The model under review builds one solid part; all positions refer to its coordinate system, in mm. A direction names the side the tool comes from. Give positions to 0.01 mm unless a question says otherwise; leave off trailing zeros. Loops run counter-clockwise (first coordinate to the right, second up) from the corner with the lowest first, then second, coordinate; pieces in that order, holes last. Notation, with made-up numbers: M -6.75,-23 L 51.25,-23 A19 ccw 51.25,-2 Z; hole C -5.5,-29 d4. An arc over 180 degrees is marked long. Return JSON: item names as keys, results as strings. Group by question number.
```python
from build123d import *

# Parameters (mm, degrees)
SKETCH1_W           = 7.9375
SKETCH1_H           = 360.02418597
SKETCH1_3_R         = 12.7
BOSS_EXTRUDE1_DEPTH = 1.5875
SCALE1_SCALE        = 0.5


with BuildPart() as part:
    # Sketch1 → Revolve1 (revolve)
    with BuildSketch(Plane.XY, mode=Mode.PRIVATE) as revolve1_sk:
        with Locations((3.96875, 206.8008909)):
            Rectangle(SKETCH1_W, SKETCH1_H)
    revolve(revolve1_sk.sketch.rotate(Axis((0, 386.812983885, 0), (0, -1, 0)), 180), axis=Axis((0, 386.812983885, 0), (0, -1, 0)))

    # Sketch1_3 → Boss-Extrude1 (add, symmetric)
    # profile 1 of 2: a face of its own
    with BuildSketch(Plane.XY):
        with BuildLine():
            Line((-7.9375, 26.788797915), (7.9375, 26.788797915))
            ThreePointArc((7.9375, 26.788797915), (0, -27.94), (-7.9375, 26.788797915))
        make_face()
        Circle(SKETCH1_3_R, mode=Mode.SUBTRACT)
    # profile 2 of 2: a face of its own
    with BuildSketch(Plane.XY):
        with BuildLine():
            Line((-7.9375, 386.812983885), (7.9375, 386.812983885))
            ThreePointArc((7.9375, 386.812983885), (0, 441.541781801), (-7.9375, 386.812983885))
        make_face()
        with Locations((0, 413.601781801)):
            Circle(SKETCH1_3_R, mode=Mode.SUBTRACT)
    extrude(amount=BOSS_EXTRUDE1_DEPTH, both=True)


with BuildPart() as part_1:
    # Scale1: scaled about (0, 206.8008909, 0)
    add(part.part.scale(SCALE1_SCALE).moved(Location((0, 103.40044545, 0))))


solid = part_1.part
```
(1) For faces 1 (the cylindrical face through (0.56, 89.44, -0.01)), 2 (the flat face through (-2.9, 109.4, -0.794)), 3 (the flat face through (0, 317, -0.794)), 4 (the flat face through (-2.9, 109.4, 0.794)), list the 3-axis set-ups (+Z, -Z, +X, -X, +Y, -Y) from which the entire face can be reached by the end or side of a thin tool; tool diameter is ignored.
(2) For probe 1 along Y at (x, z) = (0, 0.2); probe 2 along X at (y, z) = (165, 0.75); probe 3 along Z at (x, y) = (6.5, 103), list the stretches that pass through material, from the lowest coordinate up.
(3) For pin 1 (8 mm diameter, centred on x = -2.5, y = 307.5, fed in from +Z); pin 2 (2 mm diameter, centred on x = -2.5, y = 287.5, fed in from +Z); pin 3 (1.5 mm diameter, centred on y = 230.5, z = 1.5, fed in from -X); pin 4 (7.5 mm diameter, centred on x = 0, y = 103.4, fed in from -Z), all flat-tipped, find the tip position at first contact; note any pin that passes through.
(4) Add section C-C (z = 2.5). Write out the cut boundary in (x, y).
(5) Add section A-A (x = 0). Write out the cut boundary in (y, z).
(6) Mouldability with a two-part tool opening along X and no side actions: class faces 5 (the cylindrical face through (3.41, 315.56, -0.01)), 6 (the flat face through (0, 317, 0.794)), 7 (the cylindrical face through (0.86, 208.061, 3.874)) as released by +X, released by -X, zero draft, split by the parting line, or undercut.
(7) Add section B-B (y = 193). Write out the cut boundary in (x, z), and give its area (3 significant figures).
Verdict:
{
 "1": {"face 1": "+Z, -Z", "face 2": "-Z, +X, -X, -Y", "face 3": "-Z, +X, -X, +Y", "face 4": "+Z, +X, -X, -Y"},
 "2": {"probe 1": "y = 89.43 to 97.05, 109.75 to 303.85, 316.55 to 324.17", "probe 2": "x = -3.9 to 3.9", "probe 3": "z = -0.79 to 0.79"},
 "3": {"pin 1": "stops at z = 0.79", "pin 2": "stops at z = 3.67", "pin 3": "stops at x = -3.9", "pin 4": "passes through"},
 "4": {"outline": "M -3.08,116.79 L 3.08,116.79 L 3.08,296.81 L -3.08,296.81 Z"},
 "5": {"outline": "M 89.43,-0.79 L 97.05,-0.79 L 97.05,0.79 L 89.43,0.79 Z; M 109.75,-0.79 L 116.79,-0.79 L 116.79,-3.97 L 296.81,-3.97 L 296.81,-0.79 L 303.85,-0.79 L 303.85,0.79 L 296.81,0.79 L 296.81,3.97 L 116.79,3.97 L 116.79,0.79 L 109.75,0.79 Z; M 316.55,-0.79 L 324.17,-0.79 L 324.17,0.79 L 316.55,0.79 Z"},
 "6": {"face 5": "undercut", "face 6": "zero draft", "face 7": "split by the parting line"},
 "7": {"outline": "C 0,0 d7.94", "area": "49.5 mm²"}
}
